Check sheet for the modelled part. Datum: model origin and axes. Units: mm. A direction names the side the tool comes from. Give positions to 0.01 mm unless a question says otherwise; leave off trailing zeros. Loops run counter-clockwise (first coordinate to the right, second up) from the corner with the lowest first, then second, coordinate; pieces in that order, holes last. Notation, with made-up numbers: (84.25, -22) - (104.25, -22) arc R23 ccw to (104.25, 5) - close; hole circle Ø9 at (23, -15.5). An arc over 180 degrees is marked (long way). Use one line per item in the form item = value.
from build123d import *

# Parameters (mm, degrees)
F0_W     = 7.62
F0_H     = 7.62
F1_DEPTH = 9.652
F2_R     = 2.413
F3_DEPTH = 1.778
F4_W     = 6.2738
F4_H     = 6.2738
F5_DEPTH = 8.128


with BuildPart() as f1:
    # F0 (on Top) → F1 (new body)
    with BuildSketch(Plane.XY):
        Rectangle(F0_W, F0_H)
    extrude(amount=F1_DEPTH)

    # F2 (on face) → F3 (join)
    with BuildSketch(Plane.XY.offset(9.652)):
        Circle(F2_R)
    extrude(amount=F3_DEPTH)

    # F4 (on face) → F5 (cut)
    with BuildSketch(Plane(origin=(0, 0, 0), x_dir=(1, 0, 0), z_dir=(0, 0, -1))):
        Rectangle(F4_W, F4_H)
    extrude(amount=-F5_DEPTH, mode=Mode.SUBTRACT)


solid = f1.part
Item 1: Thickness scan on L1, parallel to Y at x = -1.75, z = 5; L2, parallel to Z at x = -2, y = -2. Record the ranges inside material, lowest first.
Answer block:
L1 = -3.81 to -3.14, 3.14 to 3.81
L2 = 8.13 to 9.65
Item 2: Gauge pin test, flat end, axial feed: P1, Ø3, axis at x = -1.5, y = 0.5, coming from the -Z side. Record the tip position at first contact, or that the pin passes through.
Answer block:
P1 = 8.13
Item 3: Section check C-C on x = 0. Record the boundary of the cut face in (y, z), then the cut area to 3 significant figures.
Answer block:
outline = (-3.81, 0) - (-3.14, 0) - (-3.14, 8.13) - (3.14, 8.13) - (3.14, 0) - (3.81, 0) - (3.81, 9.65) - (2.41, 9.65) - (2.41, 11.43) - (-2.41, 11.43) - (-2.41, 9.65) - (-3.81, 9.65) - close
area = 31.1 mm2
Item 4: Section check A-A on z = 3. Record the boundary of the cut face in (x, y), then the cut area to 3 significant figures.
Answer block:
outline = (-3.81, -3.81) - (3.81, -3.81) - (3.81, 3.81) - (-3.81, 3.81) - close; hole (-3.14, -3.14) - (3.14, -3.14) - (3.14, 3.14) - (-3.14, 3.14) - close
area = 18.7 mm2
Item 5: Mould release check, pull along Y, two halves, no side actions. Record for faces 4 (the face through (3.3, 0.1, 0)), 5 (the face through (-1.915, -1.468, 10.529)), 6 (the face through (0, -3.137, 4)): released by +Y, released by -Y, zero draft, split by the parting line, or undercut.
Answer block:
face_4 = zero draft
face_5 = split by the parting line
face_6 = undercut
Item 6: Access from +Z, -Z, +X, -X, +Y, -Y to the whole of each face (thin tool, end or side, straight path). Record for faces 1 (the face through (3.81, 0, 5)), 2 (the face through (-2, 2, 9.652)), 3 (the face through (0, 3.137, 4)).
Answer block:
face_1 = +Z, -Z, +X, +Y, -Y
face_2 = +Z
face_3 = -Z
Item 7: Section check B-B on y = -3. Record the boundary of the cut face in (x, z), then the cut area to 3 significant figures.
Answer block:
outline = (-3.81, 0) - (-3.14, 0) - (-3.14, 8.13) - (3.14, 8.13) - (3.14, 0) - (3.81, 0) - (3.81, 9.65) - (-3.81, 9.65) - close
area = 22.6 mm2
